Geometry check sheet. Reference: the model listing, model coordinates, mm. Face numbers are marked on the shaded views. A direction names the side the tool comes from. Give positions to 0.01 mm unless a question says otherwise; leave off trailing zeros. Write each loop counter-clockwise with the first axis right and the second up, starting at its lowest first coordinate (ties: lowest second). Pieces come first, ordered by that corner, then holes. Notation, with made-up numbers: M -12,57 L 10,57 A33 cw 10,93 Z; hole C 84.5,56.5 d5. An arc over 180 degrees is marked long. One line per item, written item: value. Start each with the question number.
1. Scan lines: line 1 (X direction, y = 59.5, z = 0); line 2 (Z direction, x = 0, y = 14). Record each from-to range of solid material in increasing order.
2. Gauge pin test, flat ends, axial feed: pin 1 (1 mm diameter, centred on x = 1, z = 46.5, fed in from -Y); pin 2 (1.5 mm diameter, centred on x = -42, z = 39.5, fed in from -Y); pin 3 (10 mm diameter, centred on y = 28, z = 30.5, fed in from -X). Record the tip position at first contact, or that the pin passes through.
3. Tool access check on the marked faces 1 and 2. Record the directions out of +Z, -Z, +X, -X, +Y, -Y that give a thin tool (end or side, any length) a straight path to the whole face; none if there is none.
4. Cross-section at A-A on x = 0. Record the cut outline in (y, z).
5. Cross-section at B-B on z = 0. Record the cut outline in (x, y), then the cut area to 3 significant figures.
6. Release check for a two-part mould opening along Z. For the marked faces 3, 4 and 5 record: pulls with the +Z half, pulls with the -Z half, needs draft (parallel to the pull), parting line crosses it, or undercut.
7. Cross-section at C-C on y = 60.5. Record the cut outline in (x, z), then the cut area to 3 significant figures.
from build123d import *

# Parameters (mm, degrees)
F2_T = -5


with BuildPart() as f1:
    # F0 (on Top) → F1 (revolve)
    with BuildSketch(Plane.XY):
        Polygon((-25.3672786057, 19.3985067308), (-25.3672786057, 0), (0, 0), (0, 66.0295262933), (-72.3713487387, 66.0295262933), (-72.3713487387, 43.6466373503), (-52.2267483175, 26.4864228666), align=None)
    revolve(axis=Axis((0, 33.0147631466, 0), (0, -1, 0)))

    # F2
    f2_openings = [f1.faces().sort_by_distance(p)[0] for p in [
        (0, 66.029526, 0),
    ]]
    offset(amount=F2_T, openings=f2_openings, kind=Kind.INTERSECTION)


solid = f1.part
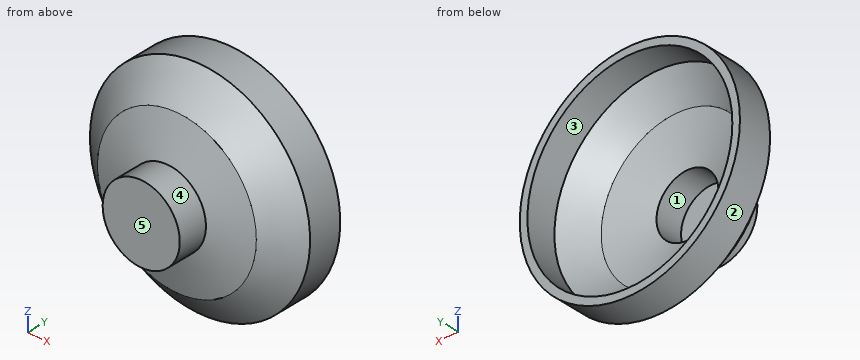
Report:
1. line 1: x = -72.37 to -67.37, 67.37 to 72.37
1. line 2: z = -25.37 to -20.37, 20.37 to 25.37
2. pin 1: stops at y = 24.85
2. pin 2: stops at y = 30.47
2. pin 3: stops at x = -52.1
3. face 1: +Y
3. face 2: +Y, -Y
4. outline: M 0,-25.37 L 19.4,-25.37 L 26.49,-52.23 L 43.65,-72.37 L 66.03,-72.37 L 66.03,-67.37 L 45.96,-67.37 L 31.03,-49.85 L 23.25,-20.37 L 5,-20.37 L 5,20.37 L 23.25,20.37 L 31.03,49.85 L 45.96,67.37 L 66.03,67.37 L 66.03,72.37 L 43.65,72.37 L 26.49,52.23 L 19.4,25.37 L 0,25.37 Z
5. outline: M -72.37,43.65 L -52.23,26.49 L -25.37,19.4 L -25.37,0 L 25.37,0 L 25.37,19.4 L 52.23,26.49 L 72.37,43.65 L 72.37,66.03 L 67.37,66.03 L 67.37,45.96 L 49.85,31.03 L 20.37,23.25 L 20.37,5 L -20.37,5 L -20.37,23.25 L -49.85,31.03 L -67.37,45.96 L -67.37,66.03 L -72.37,66.03 Z
5. area: 1,170 mm^2
6. face 3: undercut
6. face 4: parting line crosses it
6. face 5: needs draft
7. outline: C 0,0 d144.74; hole C 0,0 d134.74
7. area: 2,200 mm^2
